from build123d import *

# Parameters (mm, degrees)
SKETCH1_R           = 16
SKETCH1_R_2         = 6
BOSS_EXTRUDE1_DEPTH = 116
BOSS_EXTRUDE2_START = -6
SKETCH2_R           = 22
SKETCH2_R_2         = 6
BOSS_EXTRUDE2_DEPTH = 6
SKETCH3_R           = 22
SKETCH3_R_2         = 6
BOSS_EXTRUDE3_DEPTH = 6
BOSS_EXTRUDE4_DEPTH = 6
BOSS_EXTRUDE7_DEPTH = 3
BOSS_EXTRUDE8_DEPTH = 3
HOLE1_D             = 12
HOLE2_D             = 12


with BuildPart() as part:
    # Sketch1 → Boss-Extrude1 (new body)
    with BuildSketch(Plane(origin=(0, 0, 0), x_dir=(1, 0, 0), z_dir=(0, 1, 0))):
        with Locations(Location((0, 0, 0), (0, 0, 90))):
            Circle(SKETCH1_R)
        with Locations(Location((0, 0, 0), (0, 0, 90))):
            Circle(SKETCH1_R_2, mode=Mode.SUBTRACT)
    extrude(amount=BOSS_EXTRUDE1_DEPTH)

    # Sketch2 → Boss-Extrude2 (add)
    with BuildSketch(Plane(origin=(0, 116, 0), x_dir=(1, 0, 0), z_dir=(0, 1, 0)).offset(BOSS_EXTRUDE2_START)):
        with Locations(Location((0, 0, 0), (0, 0, 270))):
            Circle(SKETCH2_R)
        with Locations(Location((0, 0, 0), (0, 0, 90))):
            Circle(SKETCH2_R_2, mode=Mode.SUBTRACT)
    extrude(amount=BOSS_EXTRUDE2_DEPTH)

    # Sketch3 → Boss-Extrude3 (add)
    with BuildSketch(Plane.XZ):
        with Locations(Location((0, 0, 0), (0, 0, 90))):
            Circle(SKETCH3_R)
        with Locations(Location((0, 0, 0), (0, 0, 270))):
            Circle(SKETCH3_R_2, mode=Mode.SUBTRACT)
    extrude(amount=-BOSS_EXTRUDE3_DEPTH)



with BuildPart() as body_2:
    # Sketch4 → Boss-Extrude4 (new body)
    with BuildSketch(Plane(origin=(-100, 0, 0), x_dir=(0, 0, -1), z_dir=(1, 0, 0))):
        with BuildLine():
            Line((-38, 116), (38, 116))
            Line((38, 116), (38, 80))
            Line((38, 80), (17.620559303, -17.676396314))
            ThreePointArc((17.620559303, -17.676396314), (0, -32), (-17.620559303, -17.676396314))
            Line((-17.620559303, -17.676396314), (-38, 80))
            Line((-38, 80), (-38, 116))
        make_face()
    extrude(amount=BOSS_EXTRUDE4_DEPTH)


with BuildPart() as part_1:
    add(part.part)

    add(body_2.part)  # Boss-Extrude7 merges body 2
    # Sketch5 → Boss-Extrude7 (add, symmetric)
    with BuildSketch(Plane.XY):
        Polygon((-100, 116), (-21, 116), (-21, 110), (-15, 110), (-15, 6), (-21, 6), (-21, 0), (-100, 0), align=None)
    extrude(amount=BOSS_EXTRUDE7_DEPTH, both=True)

    # Sketch6 → Boss-Extrude8 (add, symmetric)
    with BuildSketch(Plane(origin=(0, 58, 0), x_dir=(1, 0, 0), z_dir=(0, 1, 0))):
        with BuildLine():
            Line((-94, 38), (-94, -38))
            Line((-94, -38), (3.580633879, -15.594199596))
            ThreePointArc((3.580633879, -15.594199596), (-16, 0), (3.580633879, 15.594199596))
            Line((3.580633879, 15.594199596), (-94, 38))
        make_face()
    extrude(amount=BOSS_EXTRUDE8_DEPTH, both=True)

    # Hole1 (through all)
    with Locations(Plane(origin=(-94, 0, 0), x_dir=(0, 0, -1), z_dir=(1, 0, 0))):
        with Locations((0, -14), (-22, 98)):
            Hole(HOLE1_D / 2)

    # Hole2 (through all)
    with Locations(Plane(origin=(-94, 0, 0), x_dir=(0, 0, -1), z_dir=(1, 0, 0))):
        with Locations((22, 98)):
            Hole(HOLE2_D / 2)


solid = part_1.part
The listing builds one solid part. Answer for the finished solid, in the listing's coordinates (mm). A direction names the side the tool comes from. Coordinates: 2 decimals unless noted, no trailing zeros. Order: outer loops, then holes, each group sorted by start corner. A loop starts at its lowest first (then second) coordinate and runs counter-clockwise, first axis right, second up.
Q1. For a pull along Z with two mould halves and no side action, classify faces 6 (the face through (15.986, 57.272, 0.661)), 7 (the face through (-97.04, 103.95, -22.78)), 8 (the face through (-97.04, 30.48, 27.67)) as pulls with the +Z half, pulls with the -Z half, needs draft (parallel to the pull), parting line crosses it, or undercut.
Q2. A cutting plane is placed at A-A, the plane y = 98. Write down the section's boundary in (x, z).
Q3. A cutting plane is placed at B-B, the plane z = 26. Write down the section's boundary in (x, y), and give its area (3 significant figures).
Q4. A cutting plane is placed at C-C, the plane x = 0. Write down the section's boundary in (y, z), and give its area (3 significant figures).
Q5. Consider line 1 (Y direction, x = -15, z = -13.5); line 2 (Z direction, x = 0, y = 37.5); line 3 (Z direction, x = -21.5, y = 109). Determine where each line is inside the solid, lowest interval first.
Q6. A cutting plane is placed at D-D, the plane y = 74.5. Write down the section's boundary in (x, z), and give its area (3 significant figures).
Q7. Given P1, Ø1, axis at x = -12.5, y = 87.5, coming from the -Z side; P2, Ø10, axis at x = -48.5, y = 97.5, coming from the -Z side; P3, Ø6, axis at y = -12, z = -3.5, coming from the +X side, each flat-ended and moving along its own axis, determine where each tip first touches the part or whether it passes through.
Q8. Which of the six approach directions +Z, -Z, +X, -X, +Y, -Y give full straight-line access (tool end or side, diameter ignored) to faces 1 (the face through (21.98, 112.96, 0.93)), 2 (the face through (-10, 0, -2)), 3 (the face through (-94, 22, 7)), 4 (the face through (-94, 58, 36)), 5 (the face through (10, 110, 13))?
Answers follow:
1. face 6: parting line crosses it
1. face 7: undercut
1. face 8: pulls with the +Z half
2. outline: (-100, -38) - (-94, -38) - (-94, -28) - (-100, -28) - close; (-100, -16) - (-94, -16) - (-94, -3) - (-15.72, -3) arc R16 ccw (long way) to (-15.72, 3) - (-94, 3) - (-94, 16) - (-100, 16) - close; (-100, 28) - (-94, 28) - (-94, 38) - (-100, 38) - close; hole circle Ø12 at (0, 0)
3. outline: (-100, 22.49) - (-94, 22.49) - (-94, 55) - (-41.74, 55) - (-41.74, 61) - (-94, 61) - (-94, 93.53) - (-100, 93.53) - close; (-100, 102.47) - (-94, 102.47) - (-94, 116) - (-100, 116) - close
3. area: 821 mm2
4. outline: (0, -22) - (6, -22) - (6, -16) - (55, -16) - (55, -16.42) - (61, -16.42) - (61, -16) - (110, -16) - (110, -22) - (116, -22) - (116, -6) - (0, -6) - close; (0, 6) - (116, 6) - (116, 22) - (110, 22) - (110, 16) - (61, 16) - (61, 16.42) - (55, 16.42) - (55, 16) - (6, 16) - (6, 22) - (0, 22) - close
4. area: 2,470 mm2
5. line 1: y = 0 to 6, 55 to 61, 110 to 116
5. line 2: z = -16 to -6, 6 to 16
5. line 3: z = -3 to 3
6. outline: (-100, -36.85) - (-94, -36.85) - (-94, -3) - (-15.72, -3) arc R16 ccw (long way) to (-15.72, 3) - (-94, 3) - (-94, 36.85) - (-100, 36.85) - close; hole circle Ø12 at (0, 0)
6. area: 1,600 mm2
7. P1: stops at z = -10.58
7. P2: stops at z = -3
7. P3: stops at x = -94
8. face 1: +Y
8. face 2: +Z, -Z, +X, -Y
8. face 3: -Y
8. face 4: +Z, -X, -Y
8. face 5: none
